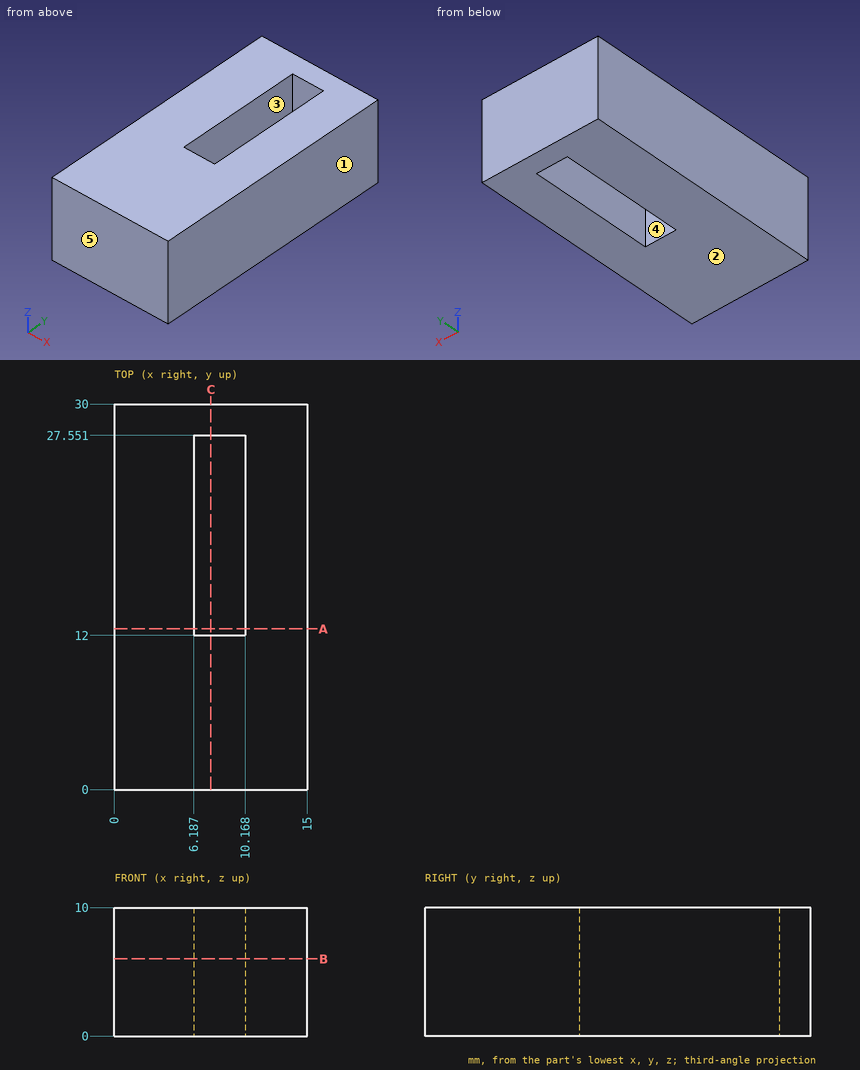
For this review, use the dimensioned drawing (mm, ordinates from the lowest corner) and the shaded views. A direction names the side the tool comes from. Give positions to 0.01 mm unless a question says otherwise; leave off trailing zeros. Order: outer loops, then holes, each group sorted by start corner. A loop starts at its lowest first (then second) coordinate and runs counter-clockwise, first axis right, second up. Notation, with made-up numbers: (88, 0.5) - (118, 0.5) arc R30 ccw to (118, 31.5) - close; hole circle Ø10 at (47, 50). An arc over 180 degrees is marked (long way). Write item = value, one per line. Start each with the question number.
Q1. Tool access review of the marked faces 4 and 5: name each direction out of +Z, -Z, +X, -X, +Y, -Y from which nothing blocks a thin tool from reaching the whole face with its end or side.
Q2. Mouldability with a two-part tool opening along X and no side actions: class the marked faces 1, 2 and 3 as released by +X, released by -X, zero draft, split by the parting line, or undercut.
Q3. We need section A-A on y = 12.5. State the section outline as (x, z) points.
Q4. To check wall thickness, follow L1, parallel to Y at x = 10, z = 4.25; L2, parallel to X at y = 21, z = 6.25. State the ranges of each line that lie inside material, in increasing order. Write a range as from..to.
Q5. We need section C-C on x = 7.5. State the section outline as (y, z) points.
Q6. We need section B-B on z = 6. State the section outline as (x, y) points, plus the area to 3 significant figures.
Working result:
q1.face_4 = +Z, -Z
q1.face_5 = +Z, -Z, +X, -X, -Y
q2.face_1 = released by +X
q2.face_2 = zero draft
q2.face_3 = undercut
q3.outline = (0, 0) - (6.19, 0) - (6.19, 10) - (0, 10) - close; (10.17, 0) - (15, 0) - (15, 10) - (10.17, 10) - close
q4.L1 = 0..12, 27.55..30
q4.L2 = 0..6.19, 10.17..15
q5.outline = (0, 0) - (12, 0) - (12, 10) - (0, 10) - close; (27.55, 0) - (30, 0) - (30, 10) - (27.55, 10) - close
q6.outline = (0, 0) - (15, 0) - (15, 30) - (0, 30) - close; hole (6.19, 12) - (10.17, 12) - (10.17, 27.55) - (6.19, 27.55) - close
q6.area = 388 mm²
